Source: CAD feature listing. Evaluate the final solid. Frame: model axes, mm. Coordinates: 2 decimals unless noted, no trailing zeros. Write each loop counter-clockwise with the first axis right and the second up, starting at its lowest first coordinate (ties: lowest second). Pieces come first, ordered by that corner, then holes. Notation, with made-up numbers: (53, 62) -> (72, 62) arc R19 ccw to (72, 74) -> close; hole circle Ø6 at (3, 76.5). An arc over 180 degrees is marked (long way). One line per item, written item: value. Start each with the question number.
1. First-contact query: P1, Ø8, axis at x = -28.5, z = -19.5, coming from the -Y side; P2, Ø5, axis at x = -25, y = 3.5, coming from the +Z side; P3, Ø1, axis at x = 18, y = 6.5, coming from the +Z side. Flat tips, straight axial feed; report the tip coordinate or a pass-through.
2. Mould query, pull axis Z, two halves, no side actions, for faces 1 (the flat face through (-11, 0, 11)), 2 (the cylindrical face through (-2.93, 1.98, 13.18)). Classes: released by +Z, released by -Z, zero draft, split by the parting line, or undercut.
3. Section query A-A, the plane z = 0. Output: boundary loops of the cut face in (x, y), and give its area (3 significant figures).
4. Section query B-B, the plane x = 0. Output: boundary loops of the cut face in (y, z), and give its area (3 significant figures).
5. Line query: line 1 (Z direction, x = -16, y = 8.25); line 2 (X direction, y = 1.8, z = 0); line 3 (Y direction, x = -19, z = 14). Output: solid intervals per line, ascending.
from build123d import *


# Not quite as in the source:
# - a fillet or chamfer that OpenCascade refuses, or shapes differently, is made with other operations: its cross-section is extruded or revolved along the edge and cut away or added


with BuildPart() as f1:
    # F0 (on Top) → F1 (revolve)
    with BuildSketch(Plane.XY):
        with BuildLine():
            Line((26, 4), (13.5, 4))
            Line((13.5, 4), (13.5, 0))
            Line((13.5, 0), (26, 0))
            ThreePointArc((26, 0), (34.3358249123, 2.0438355847), (40.7808320951, 7.7117384844))
            Line((40.7808320951, 7.7117384844), (37.5, 10))
            ThreePointArc((37.5, 10), (32.4855608855, 5.5901749694), (26, 4))
        make_face()
    revolve(axis=Axis((0, 5.3547318093, 0), (0, 1, 0)))

    # F2: chamfer of 0.5 on 5 edges, made by hand

    # F2_s1 → F2_t2 (revolve, cut)
    with BuildSketch(Plane.XY):
        Polygon((14, 4), (13.5, 3.5), (13.5, 4), align=None)
    revolve(axis=Axis((0, 4, 0), (0, 1, 0)), mode=Mode.SUBTRACT)

    # F2_s3 → F2_t4 (revolve, cut)
    with BuildSketch(Plane.XY):
        Polygon((13.5, 0.5), (14, 0), (13.5, 0), align=None)
    revolve(axis=Axis((0, 0, 0), (0, 1, 0)), mode=Mode.SUBTRACT)

    # F2_s5 → F2_t6 (revolve, cut)
    with BuildSketch(Plane.XY):
        with BuildLine():
            Line((37.9030413035, 9.7188932937), (37.2169968397, 9.608773582))
            ThreePointArc((37.2169968397, 9.608773582), (37.3560341631, 9.7974365018), (37.5, 10))
            Line((37.5, 10), (37.9030413035, 9.7188932937))
        make_face()
    revolve(axis=Axis((0, 10, 0), (0, 1, 0)), mode=Mode.SUBTRACT)

    # F2_s7 → F2_t8 (revolve, cut)
    with BuildSketch(Plane.XY):
        with BuildLine():
            Line((40.4806168806, 7.2941297957), (40.3648752289, 8.0018533277))
            Line((40.3648752289, 8.0018533277), (40.7808320951, 7.7117384844))
            ThreePointArc((40.7808320951, 7.7117384844), (40.6280870104, 7.4961241001), (40.4806168806, 7.2941297957))
        make_face()
    revolve(axis=Axis((0, 7.7117384844, 0), (0, 1, 0)), mode=Mode.SUBTRACT)


solid = f1.part
Computed values:
1. P1: stops at y = 0.58
1. P2: stops at z = 31.09
1. P3: stops at z = 36.08
2. face 1: zero draft
2. face 2: undercut
3. outline: (-40.48, 7.29) arc R18.02 ccw to (-26, 0) -> (-14, 0) -> (-13.5, 0.5) -> (-13.5, 3.5) -> (-14, 4) -> (-26, 4) arc R14.02 cw to (-37.22, 9.61) -> (-37.9, 9.72) -> (-40.36, 8) -> close; (13.5, 0.5) -> (14, 0) -> (26, 0) arc R18.02 ccw to (40.48, 7.29) -> (40.36, 8) -> (37.9, 9.72) -> (37.22, 9.61) arc R14.02 cw to (26, 4) -> (14, 4) -> (13.5, 3.5) -> close
3. area: 222 mm²
4. outline: (0, -26) arc R18.02 ccw to (7.29, -40.48) -> (8, -40.36) -> (9.72, -37.9) -> (9.61, -37.22) arc R14.02 cw to (4, -26) -> (4, -14) -> (3.5, -13.5) -> (0.5, -13.5) -> (0, -14) -> close; (0, 14) -> (0.5, 13.5) -> (3.5, 13.5) -> (4, 14) -> (4, 26) arc R14.02 cw to (9.61, 37.22) -> (9.72, 37.9) -> (8, 40.36) -> (7.29, 40.48) arc R18.02 ccw to (0, 26) -> close
4. area: 222 mm²
5. line 1: z = -36.67 to -32.31, 32.31 to 36.67
5. line 2: x = -33.85 to -13.5, 13.5 to 33.85
5. line 3: y = 0 to 4
